The listing builds one solid part. Answer for the finished solid, in the listing's coordinates (mm). Face numbers are marked on the shaded views. A direction names the side the tool comes from. Round coordinates to 2 decimals unless told otherwise and drop trailing zeros. Loops run counter-clockwise (first coordinate to the right, second up) from the corner with the lowest first, then second, coordinate; pieces in that order, holes last. Notation, with made-up numbers: (-5.75, 53) -> (29.25, 53) arc R17 ccw to (29.25, 64) -> close; hole circle Ø8 at (-10.5, 8.25). An arc over 180 degrees is marked (long way). Use a Markdown table: item, result. Add a question column.
Q1. For a pull along Y with two mould halves and no side action, classify the marked faces 3, 4, 5 and 6 as released by +Y, released by -Y, zero draft, split by the parting line, or undercut.
Q2. Section D-D on y = 22 is taken. Give the vertices of the cut face in (x, z).
Q3. Consider line 1 (Y direction, x = 5, z = 7.25); line 2 (X direction, y = 12, z = 14); line 3 (Z direction, x = 14.75, y = 20). Determine where each line is inside the solid, lowest interval first.
Q4. Section B-B on y = 46 is taken. Give the vertices of the cut face in (x, z), then the cut area to 3 significant figures.
Q5. Which of the six approach directions +Z, -Z, +X, -X, +Y, -Y give full straight-line access (tool end or side, diameter ignored) to the marked faces 1 and 2?
Q6. Section C-C on x = 15 is taken. Give the vertices of the cut face in (y, z), then the cut area to 3 significant figures.
Q7. Given pin 1 Ø7 at (x, y) = (25, 46) entering from -Z, flat-ended and moving along its own axis, determine where the tip first touches the part or whether it passes through.
Q8. Section A-A on z = 7.5 is taken. Give the vertices of the cut face in (x, y), then the cut area to 3 significant figures.
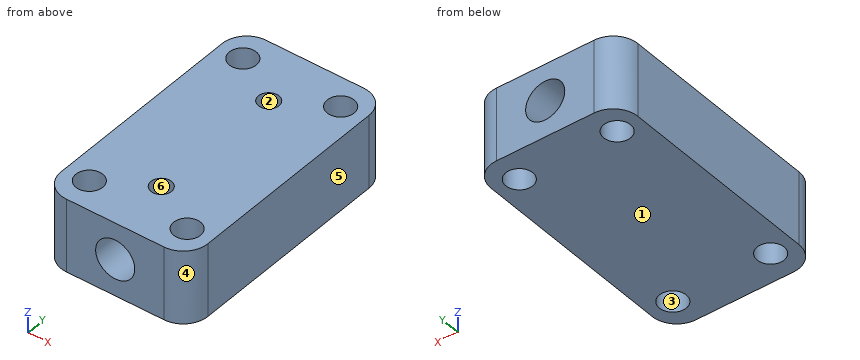
from build123d import *

# Parameters (mm, degrees)
ESQUISSE1_W                  = 30
ESQUISSE1_H                  = 52
BOSS_EXTRU_1_DEPTH           = 15
ENL_V_MAT_EXTRU_1_DEPTH      = 62.878914018
ENL_V_MAT_EXTRU_1_DEPTH_BACK = 62.878914018
ESQUISSE2_R                  = 4
ESQUISSE3_R                  = 2.75
ENL_V_MAT_EXTRU_2_DEPTH      = 62.878914018
CONG_1_R                     = 5
ESQUISSE4_R                  = 2.1
ENL_V_MAT_EXTRU_3_DEPTH      = 10


with BuildPart() as part:
    # Esquisse1 → Boss.-Extru.1 (new body)
    with BuildSketch(Plane.XY):
        with Locations((15, 26)):
            Rectangle(ESQUISSE1_W, ESQUISSE1_H)
    extrude(amount=BOSS_EXTRU_1_DEPTH)

    # Esquisse2 → Enlèv. mat.-Extru.1 (cut, two sides: drawn at the far end of the back side and taken through both)
    with BuildSketch(Plane(origin=(0, 52, 0), x_dir=(1, 0, 0), z_dir=(0, 1, 0)).offset(-ENL_V_MAT_EXTRU_1_DEPTH_BACK)):
        with Locations(Location((15, -7.5, 0), (0, 0, 270))):
            Circle(ESQUISSE2_R)
    extrude(amount=ENL_V_MAT_EXTRU_1_DEPTH + ENL_V_MAT_EXTRU_1_DEPTH_BACK, mode=Mode.SUBTRACT)

    # Esquisse3 → Enlèv. mat.-Extru.2 (cut, through all)
    with BuildSketch(Plane.XY.offset(15)):
        with Locations((5, 46)):
            Circle(ESQUISSE3_R)
        with Locations(Location((25, 46, 0), (0, 0, 180))):
            Circle(ESQUISSE3_R)
        with Locations((25, 6)):
            Circle(ESQUISSE3_R)
        with Locations(Location((5, 6, 0), (0, 0, 180))):
            Circle(ESQUISSE3_R)
    extrude(amount=-ENL_V_MAT_EXTRU_2_DEPTH, mode=Mode.SUBTRACT)

    # Congé1
    cong_1_edges = [part.edges().sort_by_distance(p)[0] for p in [
        (0, 52, 7.5),
        (30, 52, 7.5),
        (30, 0, 7.5),
        (0, 0, 7.5),
    ]]
    fillet(cong_1_edges, radius=CONG_1_R)

    # Esquisse4 → Enlèv. mat.-Extru.3 (cut)
    with BuildSketch(Plane.XY.offset(15)):
        with Locations((15, 40)):
            Circle(ESQUISSE4_R)
        with Locations(Location((15, 12, 0), (0, 0, 89.999999995))):
            Circle(ESQUISSE4_R)
    extrude(amount=-ENL_V_MAT_EXTRU_3_DEPTH, mode=Mode.SUBTRACT)


solid = part.part
Checked values:
| question | item | result |
|---|---|---|
| 1 | face 3 | undercut |
| 1 | face 4 | released by -Y |
| 1 | face 5 | zero draft |
| 1 | face 6 | undercut |
| 2 | outline | (0, 0) -> (30, 0) -> (30, 15) -> (0, 15) -> close; hole circle Ø8 at (15, 7.5) |
| 3 | line 1 | y = 0 to 3.25, 8.75 to 43.25, 48.75 to 52 |
| 3 | line 2 | x = 0 to 12.9, 17.1 to 30 |
| 3 | line 3 | z = 0 to 3.51, 11.49 to 15 |
| 4 | outline | (0, 0) -> (2.25, 0) -> (2.25, 15) -> (0, 15) -> close; (7.75, 0) -> (22.25, 0) -> (22.25, 15) -> (7.75, 15) -> close; (27.75, 0) -> (30, 0) -> (30, 15) -> (27.75, 15) -> close; hole circle Ø8 at (15, 7.5) |
| 4 | area | 235 mm2 |
| 5 | face 1 | -Z, +X, -X, +Y, -Y |
| 5 | face 2 | +Z |
| 6 | outline | (0, 0) -> (52, 0) -> (52, 3.5) -> (0, 3.5) -> close; (0, 11.5) -> (9.9, 11.5) -> (9.9, 15) -> (0, 15) -> close; (14.1, 11.5) -> (37.9, 11.5) -> (37.9, 15) -> (14.1, 15) -> close; (42.1, 11.5) -> (52, 11.5) -> (52, 15) -> (42.1, 15) -> close |
| 6 | area | 335 mm2 |
| 7 | pin 1 | stops at z = 0 |
| 8 | outline | (0, 5) arc R5 ccw to (5, 0) -> (11, 0) -> (11, 52) -> (5, 52) arc R5 ccw to (0, 47) -> close; (19, 0) -> (25, 0) arc R5 ccw to (30, 5) -> (30, 47) arc R5 ccw to (25, 52) -> (19, 52) -> close; hole circle Ø5.5 at (5, 6); hole circle Ø5.5 at (5, 46); hole circle Ø5.5 at (25, 6); hole circle Ø5.5 at (25, 46) |
| 8 | area | 1,030 mm2 |
